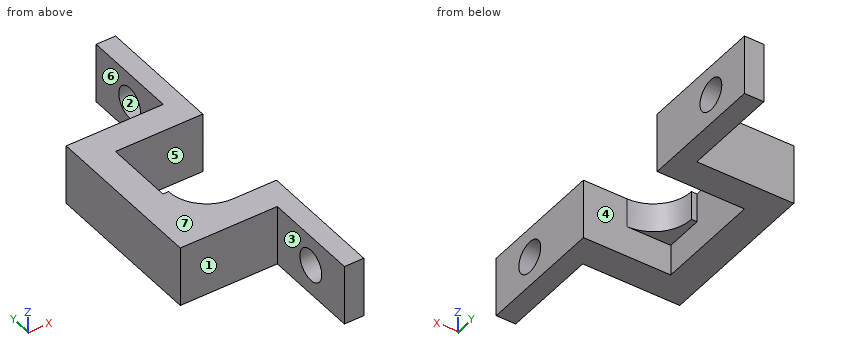
from build123d import *

# Parameters (mm, degrees)
EXTRUDE_1_DEPTH     = 3
EXTRUDE_5_DEPTH     = 3.2
SKETCH_6_W          = 2
SKETCH_6_H          = 6.2
EXTRUDE_6_DEPTH     = 10
SKETCH_7_W          = 2
SKETCH_7_H          = 6.2
EXTRUDE_7_DEPTH     = 10
CUT_EXTRUDE_1_REACH = 23.341
SKETCH_8_R          = 1.625


with BuildPart() as part:
    # 草圖1 → 填料-伸長1 (new body)
    with BuildSketch(Plane.XY):
        with BuildLine():
            Line((5.864342343, -5.42098501), (5.864342343, -8.42098501))
            Line((5.864342343, -8.42098501), (-6.135657657, -8.42098501))
            Line((-6.135657657, -8.42098501), (-6.135657657, 8.57901499))
            Line((-6.135657657, 8.57901499), (5.864342343, 8.57901499))
            Line((5.864342343, 8.57901499), (5.864342343, 5.57901499))
            Line((5.864342343, 5.57901499), (-3.135657657, 5.57901499))
            Line((-3.135657657, 5.57901499), (-3.135657657, -1.50098501))
            Line((-3.135657657, -1.50098501), (-2.555657657, -1.50098501))
            ThreePointArc((-2.555657657, -1.50098501), (-1.407516239, -4.272843593), (1.364342343, -5.42098501))
            Line((1.364342343, -5.42098501), (5.864342343, -5.42098501))
        make_face()
    extrude(amount=EXTRUDE_1_DEPTH)

    # 草圖5 → 填料-伸長5 (add)
    with BuildSketch(Plane(origin=(0, 0, 0), x_dir=(-1, 0, 0), z_dir=(0, 0, -1))):
        Polygon((3.135657657, 5.57901499), (-5.864342343, 5.57901499), (-5.864342343, 8.57901499), (6.135657657, 8.57901499), (6.135657657, -8.42098501), (-5.864342343, -8.42098501), (-5.864342343, -5.42098501), (3.135657657, -5.42098501), align=None)
    extrude(amount=EXTRUDE_5_DEPTH)

    # 草圖6 → 填料-伸長6 (add)
    with BuildSketch(Plane(origin=(0, 8.57901499, 0), x_dir=(1, 0, 0), z_dir=(0, 1, 0))):
        with Locations((4.864342343, 0.1)):
            Rectangle(SKETCH_6_W, SKETCH_6_H)
    extrude(amount=EXTRUDE_6_DEPTH)

    # 草圖7 → 填料-伸長7 (add)
    with BuildSketch(Plane.XZ.offset(8.42098501)):
        with Locations((4.864342343, -0.1)):
            Rectangle(SKETCH_7_W, SKETCH_7_H)
    extrude(amount=EXTRUDE_7_DEPTH)

    # 草圖8 → 除料-伸長1 (cut, up to next)
    with BuildSketch(Plane.ZY.offset(-3.864342343), mode=Mode.PRIVATE) as cut_extrude_1_sk1:
        with Locations(Location((-0.1, -13.42098501, 0), (0, 0, 270))):
            Circle(SKETCH_8_R)
    cut_extrude_1_tool1 = extrude(cut_extrude_1_sk1.sketch, amount=-CUT_EXTRUDE_1_REACH, mode=Mode.PRIVATE) & part.part
    # 草圖8 → 除料-伸長1 (cut, up to next)
    with BuildSketch(Plane.ZY.offset(-3.864342343), mode=Mode.PRIVATE) as cut_extrude_1_sk2:
        with Locations(Location((-0.1, 13.57901499, 0), (0, 0, 270))):
            Circle(SKETCH_8_R)
    cut_extrude_1_tool2 = extrude(cut_extrude_1_sk2.sketch, amount=-CUT_EXTRUDE_1_REACH, mode=Mode.PRIVATE) & part.part
    add(cut_extrude_1_tool1.solids().sort_by_distance((3.864342, -13.420985, -0.1))[0], mode=Mode.SUBTRACT)
    add(cut_extrude_1_tool2.solids().sort_by_distance((3.864342, 13.579015, -0.1))[0], mode=Mode.SUBTRACT)


solid = part.part
Can you work these out from the model? Positions are in its coordinate system, mm. Face numbers are marked on the shaded views. A direction names the side the tool comes from. Coordinates: 2 decimals unless noted, no trailing zeros. Write each loop counter-clockwise with the first axis right and the second up, starting at its lowest first coordinate (ties: lowest second). Pieces come first, ordered by that corner, then holes. Notation, with made-up numbers: (8.5, 37.25) -> (59.5, 37.25) arc R9 ccw to (59.5, 52.25) -> close; hole circle Ø8 at (3, 30.25). An arc over 180 degrees is marked (long way). Write item = value, one per line.
(1) Imagine slicing it at D-D (x = 0). Please give me the cut outline in (y, z).
Verdict:
outline = (-8.42, -3.2) -> (-5.42, -3.2) -> (-5.42, 0) -> (-5.18, 0) -> (-5.18, 3) -> (-8.42, 3) -> close; (5.58, -3.2) -> (8.58, -3.2) -> (8.58, 3) -> (5.58, 3) -> close
(2) For pin 1 (3 mm diameter, centred on x = 0, z = 0.5, fed in from -Y); pin 2 (3 mm diameter, centred on x = -1, y = -3, fed in from -Z); pin 3 (1.9 mm diameter, centred on y = 12.5, z = -1, fed in from -X), each with a flat end and sliding along its axis, tell me the tip position at first contact or that it passes through.
Verdict:
pin_1 = -8.42
pin_2 = 0
pin_3 = 3.86
(3) Imagine slicing it at A-A (x = 3). Please give me the cut outline in (y, z).
Verdict:
outline = (-8.42, -3.2) -> (-5.42, -3.2) -> (-5.42, 3) -> (-8.42, 3) -> close; (5.58, -3.2) -> (8.58, -3.2) -> (8.58, 3) -> (5.58, 3) -> close
(4) Thinking about a two-plate mould opening in Y: for the marked faces 1, 2, 3 and 4, which applies, +Y half, -Y half, draft (parallel to the pull), parting line (faces both ways), or undercut?
Verdict:
face_1 = -Y half
face_2 = undercut
face_3 = draft
face_4 = undercut
(5) Imagine slicing it at B-B (z = -2.5). Please give me the cut outline in (x, y).
Verdict:
outline = (-6.14, -8.42) -> (3.86, -8.42) -> (3.86, -18.42) -> (5.86, -18.42) -> (5.86, -5.42) -> (-3.14, -5.42) -> (-3.14, 5.58) -> (5.86, 5.58) -> (5.86, 18.58) -> (3.86, 18.58) -> (3.86, 8.58) -> (-6.14, 8.58) -> close
(6) Imagine slicing it at C-C (z = 0.5). Please give me the cut outline in (x, y), and give its area (3 significant figures).
Verdict:
outline = (-6.14, -8.42) -> (3.86, -8.42) -> (3.86, -11.91) -> (5.86, -11.91) -> (5.86, -5.42) -> (1.36, -5.42) arc R3.92 cw to (-2.56, -1.5) -> (-3.14, -1.5) -> (-3.14, 5.58) -> (5.86, 5.58) -> (5.86, 12.07) -> (3.86, 12.07) -> (3.86, 8.58) -> (-6.14, 8.58) -> close; (3.86, -18.42) -> (5.86, -18.42) -> (5.86, -14.93) -> (3.86, -14.93) -> close; (3.86, 15.09) -> (5.86, 15.09) -> (5.86, 18.58) -> (3.86, 18.58) -> close
area = 138 mm^2
(7) If I drill on probe 1 along Y at (x, z) = (5, 1.75); probe 2 along Y at (x, z) = (5, 1); probe 3 along Y at (x, z) = (-2.75, -1.75), over which ranges is the centre line in solid material (lowest first)?
Verdict:
probe_1 = -18.42 to -5.42, 5.58 to 18.58
probe_2 = -18.42 to -14.62, -12.22 to -5.42, 5.58 to 12.38, 14.78 to 18.58
probe_3 = -8.42 to -5.42, 5.58 to 8.58
(8) On a 3-axis mill with a long thin cutter (end or side, diameter ignored), from which of +Z, -Z, +X, -X, +Y, -Y can I reach the whole of each face in a straight line? I mean the marked faces 5, 6 and 7. Say none if no direction works.
Verdict:
face_5 = +Z, -Z, +X
face_6 = +Z, -Z, -X, +Y
face_7 = +Z, +X, -X, +Y, -Y
